Check sheet for the modelled part. Datum: model origin and axes. Units: mm. A direction names the side the tool comes from. Round coordinates to 2 decimals unless told otherwise and drop trailing zeros. Order: outer loops, then holes, each group sorted by start corner. A loop starts at its lowest first (then second) coordinate and runs counter-clockwise, first axis right, second up. Notation, with made-up numbers: (38.25, 10.25) -> (45.25, 10.25) arc R14 ccw to (45.25, 30.25) -> close; hole circle Ø4 at (24, 6). An arc over 180 degrees is marked (long way). Answer in a Markdown table with one row per item. Add a question column.
1. Sectioned sample at D-D, the plane z = 15. Record the boundary of the cut face in (x, y), then the cut area to 3 significant figures.
2. Material ranges on L1, parallel to Z at x = 0, y = 1.3; L2, parallel to Z at x = 0, y = 4.05, recorded low to high. Write a range as from..to.
3. Sectioned sample at A-A, the plane z = 0. Record the boundary of the cut face in (x, y), then the cut area to 3 significant figures.
4. Depth check by flat-ended pin: P1, Ø1.5, axis at x = 20.5, y = 2, coming from the +Z side; P2, Ø2, axis at x = -14.5, y = 2.5, coming from the -Z side; P3, Ø1, axis at x = 19, y = 1.5, coming from the -Z side. Enter the tip coordinate at first touch or a pass-through.
5. Access from +Z, -Z, +X, -X, +Y, -Y to the whole of each face (thin tool, end or side, straight path). Record for faces 1 (the flat face through (-11, 3, -24)), 2 (the cylindrical face through (0, 2, 32)).
6. Draft check along Z on faces 3 (the flat face through (-0.6, 5, 29.4)), 4 (the cylindrical face through (20.765, 2.465, 39.923)), 5 (the cylindrical face through (32, 2, 0)). Enter one of: +Z half, -Z half, draft (parallel to the pull), parting line (faces both ways), or undercut.
7. Sectioned sample at C-C, the plane x = 0. Record the boundary of the cut face in (y, z).
8. Sectioned sample at B-B, the plane y = 3.9. Record the boundary of the cut face in (x, z), then the cut area to 3 significant figures.
```python
from build123d import *

# Parameters (mm, degrees)
SKETCH_1_R         = 45
SKETCH_1_R_2       = 3
SKETCH_1_R_3       = 23
EXTRUDE_3_DEPTH    = 5
SKETCH1_R          = 29
SKETCH1_R_2        = 26
CUT_EXTRUDE1_DEPTH = 2


with BuildPart() as part:
    # 草圖1 → 填料-伸長3 (new body)
    with BuildSketch(Plane(origin=(0, 0, 0), x_dir=(1, 0, 0), z_dir=(0, 1, 0))):
        Circle(SKETCH_1_R)
        with Locations((-35, 0)):
            Circle(SKETCH_1_R_2, mode=Mode.SUBTRACT)
        with Locations((35, 0)):
            Circle(SKETCH_1_R_2, mode=Mode.SUBTRACT)
        with Locations((0, -35)):
            Circle(SKETCH_1_R_2, mode=Mode.SUBTRACT)
        with Locations((0, 35)):
            Circle(SKETCH_1_R_2, mode=Mode.SUBTRACT)
        Circle(SKETCH_1_R_3, mode=Mode.SUBTRACT)
    extrude(amount=EXTRUDE_3_DEPTH)

    # Sketch1 → Cut-Extrude1 (cut)
    with BuildSketch(Plane(origin=(0, 5, 0), x_dir=(1, 0, 0), z_dir=(0, 1, 0))):
        Circle(SKETCH1_R)
        Circle(SKETCH1_R_2, mode=Mode.SUBTRACT)
    extrude(amount=-CUT_EXTRUDE1_DEPTH, mode=Mode.SUBTRACT)


solid = part.part
```
Answer key:
| question | item | result |
|---|---|---|
| 1 | outline | (-42.43, 0) -> (-17.44, 0) -> (-17.44, 5) -> (-21.24, 5) -> (-21.24, 3) -> (-24.82, 3) -> (-24.82, 5) -> (-42.43, 5) -> close; (17.44, 0) -> (42.43, 0) -> (42.43, 5) -> (24.82, 5) -> (24.82, 3) -> (21.24, 3) -> (21.24, 5) -> (17.44, 5) -> close |
| 1 | area | 236 mm² |
| 2 | L1 | z = -45..-38, -32..-23, 23..32, 38..45 |
| 2 | L2 | z = -45..-38, -32..-29, -26..-23, 23..26, 29..32, 38..45 |
| 3 | outline | (-45, 0) -> (-38, 0) -> (-38, 5) -> (-45, 5) -> close; (-32, 0) -> (-23, 0) -> (-23, 5) -> (-26, 5) -> (-26, 3) -> (-29, 3) -> (-29, 5) -> (-32, 5) -> close; (23, 0) -> (32, 0) -> (32, 5) -> (29, 5) -> (29, 3) -> (26, 3) -> (26, 5) -> (23, 5) -> close; (38, 0) -> (45, 0) -> (45, 5) -> (38, 5) -> close |
| 3 | area | 148 mm² |
| 4 | P1 | stops at z = 40.43 |
| 4 | P2 | stops at z = -42.93 |
| 4 | P3 | stops at z = -41.02 |
| 5 | face 1 | +Y |
| 5 | face 2 | +Y, -Y |
| 6 | face 3 | draft |
| 6 | face 4 | parting line |
| 6 | face 5 | undercut |
| 7 | outline | (0, -45) -> (5, -45) -> (5, -38) -> (0, -38) -> close; (0, -32) -> (5, -32) -> (5, -29) -> (3, -29) -> (3, -26) -> (5, -26) -> (5, -23) -> (0, -23) -> close; (0, 23) -> (5, 23) -> (5, 26) -> (3, 26) -> (3, 29) -> (5, 29) -> (5, 32) -> (0, 32) -> close; (0, 38) -> (5, 38) -> (5, 45) -> (0, 45) -> close |
| 8 | outline | circle Ø90 at (0, 0); circle Ø52 at (0, 0); hole circle Ø6 at (-35, 0); hole circle Ø58 at (0, 0); hole circle Ø46 at (0, 0); hole circle Ø6 at (0, -35); hole circle Ø6 at (0, 35); hole circle Ø6 at (35, 0) |
| 8 | area | 4,070 mm² |
